from build123d import *

# Parameters (mm, degrees)
SKETCH2_R           = 1.5
BOSS_EXTRUDE1_DEPTH = 3


with BuildPart() as part:
    # Sketch2 → Boss-Extrude1 (new body)
    with BuildSketch(Plane.XY):
        with BuildLine():
            Line((-22, 3), (0, 3))
            ThreePointArc((0, 3), (1.720729309, 2.457456133), (2.819077862, 1.02606043))
            Line((2.819077862, 1.02606043), (5.213218866, -5.551787916))
            ThreePointArc((5.213218866, -5.551787916), (4.604366119, -8.606371192), (1.613091911, -9.474391512))
            Line((1.613091911, -9.474391512), (-22.781049092, -2.896543167))
            ThreePointArc((-22.781049092, -2.896543167), (-24.974023327, 0.393935591), (-22, 3))
        make_face()
        with Locations((-22, 0)):
            Circle(SKETCH2_R, mode=Mode.SUBTRACT)
        Circle(SKETCH2_R, mode=Mode.SUBTRACT)
        with Locations((2.394141003, -6.577848346)):
            Circle(SKETCH2_R, mode=Mode.SUBTRACT)
    extrude(amount=BOSS_EXTRUDE1_DEPTH)


solid = part.part
Input: part model. Units: mm. Frame: model coordinates. Coordinates: 2 decimals unless noted, no trailing zeros. Loops run counter-clockwise (first coordinate to the right, second up) from the corner with the lowest first, then second, coordinate; pieces in that order, holes last.
(1) Material intervals for probe 1 along X at (y, z) = (0.75, 2.95); probe 2 along X at (y, z) = (0.25, 2.3); probe 3 along Y at (x, z) = (-23, 1.7), sorted ascending.
(2) Section D-D on x = -15. Return the cut outline in (y, z).
(3) Pull-direction query (Y, two-part tool) for faces 1 (the face through (-1.5, 0.07, 1.48)), 2 (the face through (1.7, 2.47, 1.48)), 3 (the face through (-10, -2, 0)); classes: released by +Y, released by -Y, zero draft, split by the parting line, or undercut.
(4) First-contact query: pin 1 Ø1 at (x, z) = (-16.5, 1) entering from -Y; pin 2 Ø3.5 at (x, y) = (0, 0) entering from +Z. Flat tips, straight axial feed; report the tip coordinate or a pass-through.
(5) Section A-A on x = 0.5. Return the cut outline in (y, z), then the cut area to 3 significant figures.
(6) Section C-C on z = 1.9. Return the cut outline in (x, y).
(7) Section B-B on y = 0. Return the cut outline in (x, z).
Data:
1. probe 1: x = -24.9 to -23.3, -20.7 to -1.3, 1.3 to 2.92
1. probe 2: x = -24.99 to -23.48, -20.52 to -1.48, 1.48 to 3.1
1. probe 3: y = -2.83 to -1.12, 1.12 to 2.83
2. outline: (-4.99, 0) - (3, 0) - (3, 3) - (-4.99, 3) - close
3. face 1: undercut
3. face 2: released by +Y
3. face 3: zero draft
4. pin 1: stops at y = -4.73
4. pin 2: stops at z = 3
5. outline: (-9.17, 0) - (-1.41, 0) - (-1.41, 3) - (-9.17, 3) - close; (1.41, 0) - (2.96, 0) - (2.96, 3) - (1.41, 3) - close
5. area: 27.9 mm2
6. outline: (-22.78, -2.9) - (1.61, -9.47) arc R3 ccw to (5.21, -5.55) - (2.82, 1.03) arc R3 ccw to (0, 3) - (-22, 3) arc R3 ccw to start; hole circle Ø3 at (-22, 0); hole circle Ø3 at (0, 0); hole circle Ø3 at (2.39, -6.58)
7. outline: (-25, 0) - (-23.5, 0) - (-23.5, 3) - (-25, 3) - close; (-20.5, 0) - (-1.5, 0) - (-1.5, 3) - (-20.5, 3) - close; (1.5, 0) - (3.19, 0) - (3.19, 3) - (1.5, 3) - close
